from build123d import *

# Parameters (mm, degrees)
BOSS_EXTRUDE1_DEPTH = 7
FILLET1_R           = 8.5
FILLET2_R           = 5.5
FILLET3_R           = 13.5
SKETCH3_W           = 27
SKETCH3_H           = 13.5
CUT_EXTRUDE1_DEPTH  = 1.8
CUT_EXTRUDE5_REACH  = 37.882
SKETCH12_W          = 12
SKETCH12_H          = 13.5
CUT_EXTRUDE6_REACH  = 37.882
SKETCH13_R          = 1.1
SKETCH17_R          = 2.1
CUT_EXTRUDE14_DEPTH = 4
FILLET4_R           = 3
SHELL2_START        = 3
SHELL2_DEPTH        = 4
SHELL2_START_2      = 4.8
SHELL2_2_DEPTH      = 2.2
SKETCH18_W          = 22
SKETCH18_H          = 22
BOSS_EXTRUDE2_DEPTH = 10
SKETCH19_W          = 18
SKETCH19_H          = 18
CUT_EXTRUDE15_DEPTH = 10
SKETCH20_R          = 5
CUT_EXTRUDE16_DEPTH = 3


# Read off the part's stored shape, not the designer's step: Shell2
with BuildPart() as part:
    # Sketch2 → Boss-Extrude1 (new body)
    with BuildSketch(Plane(origin=(0, 0, 0), x_dir=(0, 0, -1), z_dir=(1, 0, 0))):
        Polygon((-13.5, -17.5), (13.5, -17.5), (13.5, 17.5), (5.5, 32.5), (-5.5, 32.5), (-13.5, 17.5), align=None)
    extrude(amount=BOSS_EXTRUDE1_DEPTH)

    # Fillet1
    fillet1_edges = [part.edges().sort_by_distance(p)[0] for p in [
        (3.5, 32.5, 5.5),
        (3.5, 32.5, -5.5),
    ]]
    fillet(fillet1_edges, radius=FILLET1_R)

    # Fillet2
    fillet2_edges = [part.edges().sort_by_distance(p)[0] for p in [
        (3.5, 17.5, -13.5),
        (3.5, 17.5, 13.5),
    ]]
    fillet(fillet2_edges, radius=FILLET2_R)

    # Fillet3
    fillet3_edges = [part.edges().sort_by_distance(p)[0] for p in [
        (3.5, -17.5, 13.5),
        (3.5, -17.5, -13.5),
    ]]
    fillet(fillet3_edges, radius=FILLET3_R - 0.0001)  # a hair under: the kernel refuses the full size

    # Sketch3 → Cut-Extrude1 (cut)
    with BuildSketch(Plane.ZY):
        with Locations((0, -10.75)):
            Rectangle(SKETCH3_W, SKETCH3_H)
    extrude(amount=-CUT_EXTRUDE1_DEPTH, mode=Mode.SUBTRACT)

    # Sketch12 → Cut-Extrude5 (cut, up to next)
    with BuildSketch(Plane(origin=(7, 0, 0), x_dir=(0, 0, -1), z_dir=(1, 0, 0)), mode=Mode.PRIVATE) as cut_extrude5_sk1:
        with Locations((0, -10.75)):
            Rectangle(SKETCH12_W, SKETCH12_H)
    cut_extrude5_tool1 = extrude(cut_extrude5_sk1.sketch, amount=-CUT_EXTRUDE5_REACH, mode=Mode.PRIVATE) & part.part
    add(cut_extrude5_tool1.solids().sort_by_distance((7, -10.75, 0))[0], mode=Mode.SUBTRACT)

    # Sketch13 → Cut-Extrude6 (cut, up to next)
    with BuildSketch(Plane.ZY, mode=Mode.PRIVATE) as cut_extrude6_sk1:
        with Locations((-7.5, 23.5)):
            Circle(SKETCH13_R)
    cut_extrude6_tool1 = extrude(cut_extrude6_sk1.sketch, amount=-CUT_EXTRUDE6_REACH, mode=Mode.PRIVATE) & part.part
    # Sketch13 → Cut-Extrude6 (cut, up to next)
    with BuildSketch(Plane.ZY, mode=Mode.PRIVATE) as cut_extrude6_sk2:
        with Locations((-10, -8.5)):
            Circle(SKETCH13_R)
    cut_extrude6_tool2 = extrude(cut_extrude6_sk2.sketch, amount=-CUT_EXTRUDE6_REACH, mode=Mode.PRIVATE) & part.part
    # Sketch13 → Cut-Extrude6 (cut, up to next)
    with BuildSketch(Plane.ZY, mode=Mode.PRIVATE) as cut_extrude6_sk3:
        with Locations((10, -8.5)):
            Circle(SKETCH13_R)
    cut_extrude6_tool3 = extrude(cut_extrude6_sk3.sketch, amount=-CUT_EXTRUDE6_REACH, mode=Mode.PRIVATE) & part.part
    # Sketch13 → Cut-Extrude6 (cut, up to next)
    with BuildSketch(Plane.ZY, mode=Mode.PRIVATE) as cut_extrude6_sk4:
        with Locations((7.5, 23.5)):
            Circle(SKETCH13_R)
    cut_extrude6_tool4 = extrude(cut_extrude6_sk4.sketch, amount=-CUT_EXTRUDE6_REACH, mode=Mode.PRIVATE) & part.part
    add(cut_extrude6_tool1.solids().sort_by_distance((0, 23.5, -7.5))[0], mode=Mode.SUBTRACT)
    add(cut_extrude6_tool2.solids().sort_by_distance((0, -8.5, -10))[0], mode=Mode.SUBTRACT)
    add(cut_extrude6_tool3.solids().sort_by_distance((0, -8.5, 10))[0], mode=Mode.SUBTRACT)
    add(cut_extrude6_tool4.solids().sort_by_distance((0, 23.5, 7.5))[0], mode=Mode.SUBTRACT)

    # Sketch17 → Cut-Extrude14 (cut)
    with BuildSketch(Plane.ZY):
        with Locations((-7.5, 23.5)):
            Circle(SKETCH17_R)
        with Locations((7.5, 23.5)):
            Circle(SKETCH17_R)
        with Locations((-10, -8.5)):
            Circle(SKETCH17_R)
        with Locations((10, -8.5)):
            Circle(SKETCH17_R)
    extrude(amount=-CUT_EXTRUDE14_DEPTH, mode=Mode.SUBTRACT)

    # Fillet4
    fillet4_edges = [part.edges().sort_by_distance(p)[0] for p in [
        (4.4, -16.093424605, -6),
        (4.4, -16.093424605, 6),
    ]]
    fillet(fillet4_edges, radius=FILLET4_R)

    # Shell2 outline → Shell2 (cut)
    with BuildSketch(Plane.YZ.offset(SHELL2_START)):
        with BuildLine():
            Line((17.301470588, -10.205882353), (18.775176121, -9.419906069))
            ThreePointArc((18.775176121, -9.419906069), (21.033978224, -3.035838645), (27.640649185, -4.522580929))
            ThreePointArc((27.640649185, -4.522580929), (29.013659867, -2.661241858), (29.5, -0.4))
            Line((29.5, -0.4), (29.5, 0.4))
            ThreePointArc((29.5, 0.4), (29.013659867, 2.661241858), (27.640649185, 4.522580929))
            ThreePointArc((27.640649185, 4.522580929), (21.033978224, 3.035838645), (18.775176121, 9.419906069))
            Line((18.775176121, 9.419906069), (17.301470588, 10.205882353))
            ThreePointArc((17.301470588, 10.205882353), (16.731339062, 10.42535625), (16.125, 10.5))
            Line((16.125, 10.5), (-1, 10.5))
            Line((-1, 10.5), (-1, -10.5))
            Line((-1, -10.5), (16.125, -10.5))
            ThreePointArc((16.125, -10.5), (16.731339062, -10.42535625), (17.301470588, -10.205882353))
        make_face()
    extrude(amount=SHELL2_DEPTH, mode=Mode.SUBTRACT)

    # Shell2 2 outline → Shell2 2 (cut)
    with BuildSketch(Plane.YZ.offset(SHELL2_START_2)):
        with BuildLine():
            Line((-3.424568984, -10.5), (-1, -10.5))
            Line((-1, -10.5), (-1, -9))
            Line((-1, -9), (-3.4990001, -9))
            ThreePointArc((-3.4990001, -9), (-3.406267086, -9.747245183), (-3.424568984, -10.5))
        make_face()
        with BuildLine():
            Line((-3.4990001, 9), (-1, 9))
            Line((-1, 9), (-1, 10.5))
            Line((-1, 10.5), (-3.424568984, 10.5))
            ThreePointArc((-3.424568984, 10.5), (-3.406267086, 9.747245183), (-3.4990001, 9))
        make_face()
    extrude(amount=SHELL2_2_DEPTH, mode=Mode.SUBTRACT)

    # Sketch18 → Boss-Extrude2 (add)
    with BuildSketch(Plane.ZY):
        with Locations((0, 7)):
            Rectangle(SKETCH18_W, SKETCH18_H)
    extrude(amount=BOSS_EXTRUDE2_DEPTH)

    # Sketch19 → Cut-Extrude15 (cut)
    with BuildSketch(Plane.ZY.offset(10)):
        with Locations((0, 7)):
            Rectangle(SKETCH19_W, SKETCH19_H)
    extrude(amount=-CUT_EXTRUDE15_DEPTH, mode=Mode.SUBTRACT)

    # Sketch20 → Cut-Extrude16 (cut)
    with BuildSketch(Plane.ZY):
        with Locations((0, 7)):
            Circle(SKETCH20_R)
    extrude(amount=-CUT_EXTRUDE16_DEPTH, mode=Mode.SUBTRACT)


solid = part.part
Input: part model. Units: mm. Frame: model coordinates. A direction names the side the tool comes from. Round coordinates to 2 decimals unless told otherwise and drop trailing zeros. Loops run counter-clockwise (first coordinate to the right, second up) from the corner with the lowest first, then second, coordinate; pieces in that order, holes last. Notation, with made-up numbers: M 78,-34.75 L 92,-34.75 A17 cw 92,-14.75 Z; hole C 86.5,-33 d6. An arc over 180 degrees is marked long. Answer as CSV lines item,"result". Start each with the question number.
(1) Section D-D, the plane y = -8.5. Output: boundary loops of the cut face in (x, z), plus the area to 3 significant figures.
(2) Section C-C, the plane x = -1.5. Output: boundary loops of the cut face in (y, z), plus the area to 3 significant figures.
(3) Draft query along Z for faces 5 (the flat face through (-5, 7, 11)), 6 (the flat face through (0, 3, -4)), 7 (the flat face through (1.8, -7, -8)), 8 (the cylindrical face through (3.549, 31.255, -4.828)). Return one class per face: released by +Z, released by -Z, zero draft, split by the parting line, or undercut.
(4) Line query: line 1 (Y direction, x = -2.5, z = 2.5); line 2 (Z direction, x = -3.25, y = 1); line 3 (Y direction, x = 3.4, z = 10). Output: solid intervals per line, ascending. Write a range as [from, to].
(5) Reachability of faces 1 (the flat face through (3, 14, 0)), 2 (the flat face through (1.8, -6, 10)), 3 (the flat face through (-5, 18, 0)), 4 (the flat face through (4, 22.6, 8.4)) from +Z, -Z, +X, -X, +Y, -Y: full face, straight path, thin tool, end or side. Return the list, or none.
(6) First-contact query: pin 1 (6 mm diameter, centred on y = -9.5, z = 11.5, fed in from -X); pin 2 (14.5 mm diameter, centred on y = 11, z = -0.5, fed in from -X); pin 3 (1 mm diameter, centred on y = 0.5, z = -4, fed in from +X); pin 4 (3 mm diameter, centred on x = -2.5, z = 7.5, fed in from -Y). Flat tips, straight axial feed; report the tip coordinate or a pass-through.
(7) Section B-B, the plane y = 23.5. Output: boundary loops of the cut face in (x, z).
(8) Section A-A, the plane x = 2.25. Output: boundary loops of the cut face in (y, z) (3 decimals), plus the area to 3 significant figures.
Values found:
1,outline,"M 1.8,-12.73 L 7,-12.73 L 7,-11.1 L 4,-11.1 L 4,-12.1 L 1.8,-12.1 Z; M 1.8,-7.9 L 4,-7.9 L 4,-8.9 L 7,-8.9 L 7,-6 L 1.8,-6 Z; M 1.8,6 L 7,6 L 7,8.9 L 4,8.9 L 4,7.9 L 1.8,7.9 Z; M 1.8,12.1 L 4,12.1 L 4,11.1 L 7,11.1 L 7,12.73 L 1.8,12.73 Z"
1,area,"38.3 mm²"
2,outline,"M -4,-11 L 18,-11 L 18,11 L -4,11 Z; hole M -2,-9 L 16,-9 L 16,9 L -2,9 Z"
2,area,"160 mm²"
3,face 5,"released by +Z"
3,face 6,"undercut"
3,face 7,"zero draft"
3,face 8,"released by -Z"
4,line 1,"y = [-4, -2], [16, 18]"
4,line 2,"z = [-11, -9], [9, 11]"
4,line 3,"y = [-12.24, -10.6], [-6.4, -1], [17.69, 24.06]"
5,face 1,"+X"
5,face 2,"+Z, -Z, -X, -Y"
5,face 3,"+Z, -Z, -X, +Y"
5,face 4,"-X"
6,pin 1,"stops at x = 1.8"
6,pin 2,"stops at x = -10"
6,pin 3,"stops at x = 3"
6,pin 4,"stops at y = -4"
7,outline,"M 0,-10.3 L 7,-10.3 L 7,-8.6 L 4,-8.6 L 4,-9.6 L 0,-9.6 Z; M 0,-5.4 L 4,-5.4 L 4,-6.4 L 7,-6.4 L 7,-2.4 L 3,-2.4 L 3,2.4 L 7,2.4 L 7,6.4 L 4,6.4 L 4,5.4 L 0,5.4 Z; M 0,9.6 L 4,9.6 L 4,8.6 L 7,8.6 L 7,10.3 L 0,10.3 Z"
8,outline,"M -10.954,-11.571 A13.5 ccw -4,-13.5 L 16.125,-13.5 A5.5 ccw 18.713,-12.853 L 28,-7.9 A8.5 ccw 32.5,-0.4 L 32.5,0.4 A8.5 ccw 28,7.9 L 18.713,12.853 A5.5 ccw 16.125,13.5 L -4,13.5 A13.5 ccw -10.954,11.571 A3 ccw -9.408,6 L -4,6 L -4,-6 L -9.408,-6 A3 ccw Z; hole C -8.5,-10 d4.2; hole C -8.5,10 d4.2; hole C 7,0 d10; hole C 23.5,-7.5 d4.2; hole C 23.5,7.5 d4.2"
8,area,"828 mm²"
